from build123d import *

# Parameters (mm, degrees)
F1_R     = 21
F1_R_2   = 19
F3_DEPTH = 100
F4_DEPTH = 50
F7_DEPTH = 100


with BuildPart() as f2:
    # F2: sweep along a path in F0
    with BuildLine(Plane.YZ) as f2_path:
        ThreePointArc((0, -80), (-56.5685424949, -56.5685424949), (-80, 0))
    # F1 (on Top) → F2 (sweep)
    with BuildSketch(Plane.XY):
        with Locations((0, -80.018363893)):
            Circle(F1_R)
        with Locations((0, -80.018363893)):
            Circle(F1_R_2, mode=Mode.SUBTRACT)
    sweep(path=f2_path.line)

    # F3 (add): a face of the model
    f3_faces = [f2.faces().sort_by_distance(p)[0] for p in [
        (-20.4060303038, -80.018363893, 0),
    ]]
    extrude(f3_faces, amount=F3_DEPTH)

    # F4 (add): a face of the model
    f4_faces = [f2.faces().sort_by_distance(p)[0] for p in [
        (-20.4060303038, 0, -80.018363893),
    ]]
    extrude(f4_faces, amount=F4_DEPTH)


with BuildPart() as f7:
    # F6 (on face) → F7 (new body, symmetric)
    with BuildSketch(Plane.XY.offset(-80.018363893)):
        Polygon((-30.8902455139, -150), (-6.3333333333, 50), (-19, 50), (-50, 50), (-50, -150), align=None)
    extrude(amount=F7_DEPTH, both=True)


with BuildPart() as f8_1:
    # F8: instance of F7
    add(f7.part.mirror(Plane.YZ))


with BuildPart() as f2_1:
    add(f2.part)

    # F9: cut F8_1, F7
    add(f8_1.part, mode=Mode.SUBTRACT)
    add(f7.part, mode=Mode.SUBTRACT)


solid = f2_1.part
Verification items for the finished model (mm, model axes). A direction names the side the tool comes from. Round coordinates to 2 decimals unless told otherwise and drop trailing zeros. Write each loop counter-clockwise with the first axis right and the second up, starting at its lowest first coordinate (ties: lowest second). Pieces come first, ordered by that corner, then holes.
(1) Section check B-B (y = 25). Enter the section's corners in (x, z), plus the area to 3 significant figures.
Returned:
outline: (-9.4, -98.8) arc R21 ccw to (9.4, -98.8) - (9.4, -96.53) arc R19 cw to (-9.4, -96.53) - close; (-9.4, -63.51) arc R19 cw to (9.4, -63.51) - (9.4, -61.24) arc R21 ccw to (-9.4, -61.24) - close
area: 78.3 mm2
(2) Mould release check, pull along X, two halves, no side actions. Record for faces 4 (the cylindrical face through (-0.19, 19.09, -61.02)), 5 (the flat face through (-15.874, -27.704, -61.195)), 6 (the cylindrical face through (0.19, 19.094, -99.017)), 7 (the cylindrical face through (-15.48, -94.21, 49.3)): pulls with the +X half, pulls with the -X half, needs draft (parallel to the pull), parting line crosses it, or undercut.
Returned:
face 4: undercut
face 5: pulls with the -X half
face 6: undercut
face 7: parting line crosses it
(3) Depth check by flat-ended pin: pin 1 Ø3 at (x, y) = (-16, -27) entering from +Z; pin 2 Ø6 at (x, z) = (2, -31.5) entering from -Y; pin 3 Ø8 at (x, z) = (7.5, 47.5) entering from +Y. Enter the tip coordinate at first touch or a pass-through.
Returned:
pin 1: stops at z = -58.79
pin 2: stops at y = -96.85
pin 3: stops at y = -59.31
(4) Material ranges on line 1 (Y direction, x = 0, z = 54); line 2 (Y direction, x = -12.5, z = 25), recorded low to high.
Returned:
line 1: y = -101.02 to -99.02, -61.02 to -59.02
line 2: y = -96.89 to -94.33, -65.71 to -63.14
(5) Section check D-D (z = 32.5). Enter the section's corners in (x, y), plus the area to 3 significant figures.
Returned:
outline: circle Ø42 at (0, -80.02); hole circle Ø38 at (0, -80.02)
area: 251 mm2
(6) Section check C-C (x = -15.5). Enter the section's corners in (y, z).
Returned:
outline: (-94.19, 0) arc R94.19 ccw to (-24.66, -90.9) - (-24.66, -87.6) arc R91.01 cw to (-91.01, 0) - (-91.01, 100) - (-94.19, 100) - close; (-69.03, 0) arc R69.03 ccw to (-24.66, -64.48) - (-24.66, -61.06) arc R65.85 cw to (-65.85, 0) - (-65.85, 100) - (-69.03, 100) - close
(7) Access from +Z, -Z, +X, -X, +Y, -Y to the whole of each face (thin tool, end or side, straight path). Record for faces 1 (the cylindrical face through (-0.19, 19.09, -59.02)), 2 (the cylindrical face through (-15.08, -68.46, 49.3)), 3 (the cylindrical face through (0.187, 19.094, -101.018)).
Returned:
face 1: +Z, +Y
face 2: +Z
face 3: -Z, +Y, -Y
(8) Section check A-A (x = 0). Enter the section's corners in (y, z), plus the area to 3 significant figures.
Returned:
outline: (-101.02, 0) arc R101.02 ccw to (0, -101.02) - (50, -101.02) - (50, -99.02) - (0, -99.02) arc R99.02 cw to (-99.02, 0) - (-99.02, 100) - (-101.02, 100) - close; (-61.02, 0) arc R61.02 ccw to (0, -61.02) - (50, -61.02) - (50, -59.02) - (0, -59.02) arc R59.02 cw to (-59.02, 0) - (-59.02, 100) - (-61.02, 100) - close
area: 1,100 mm2
